from build123d import *

# Parameters (mm, degrees)
BOSS_EXTRUDE1_DEPTH             = 9.525
F_70_0_028_DIAMETER_HOLE1_D     = 0.7112
F_70_0_028_DIAMETER_HOLE1_DEPTH = 2.413
F_70_0_028_DIAMETER_HOLE1_TIP   = 0.213666036
FILLET5_R                       = 6.35
SKETCH90_W                      = 3.175
SKETCH90_H                      = 34.29
CUT_EXTRUDE5_DEPTH              = 49.230860727


with BuildPart() as part:
    # Sketch3 → Boss-Extrude1 (new, symmetric)
    with BuildSketch(Plane.XY):
        Polygon((0, 0), (0, 44.45), (-8.89, 44.45), (-11.43, 44.45), (-11.43, 40.64), (-8.89, 38.1), (-8.89, 16.68503416), (-16.114831723, 4.17125854), (-8.89, 0), align=None)
    extrude(amount=BOSS_EXTRUDE1_DEPTH, both=True)

    # Sketch5 → UPCHURCH 6-32 CONE (revolve, cut)
    with BuildSketch(Plane(origin=(-4.445, 25.259183771, 8.769011984), x_dir=(0, -0.8515022287907943, 0.52435098394521), z_dir=(-1, 0, 0))):
        Polygon((15.292959977, -18.808573968), (15.757749291, -16.067720643), (16.864704876, -14.270117175), (16.687021127, -14.160700376), (16.599421786, -13.998522648), (17.024527056, -14.010579296), (17.217736651, -13.696823041), (17.015625379, -13.322642754), (17.440730649, -13.334699402), (17.633940244, -13.020943147), (17.431828973, -12.64676286), (17.856934243, -12.658819508), (18.050143838, -12.345063253), (17.848032566, -11.970882966), (18.273137836, -11.982939614), (18.466347431, -11.669183359), (18.26423616, -11.295003072), (18.68934143, -11.30705972), (18.498219672, -10.503286273), (20.17440181, -11.535471185), (15.113366113, -19.754170697), (14.821385998, -19.574370744), align=None)
    upchurch_6_32_cone = revolve(axis=Axis((-4.445, 2.032, -2.119740469), (0, 0, 1)), mode=Mode.SUBTRACT)

    # Mirror1: UPCHURCH 6-32 CONE across plane
    add(upchurch_6_32_cone.mirror(Plane.XY), mode=Mode.SUBTRACT)

    # Sketch52 → UPCHURCH 10-32 CONE (revolve, cut)
    with BuildSketch(Plane(origin=(-19.421374868, 2.468387248, 20.886307367), x_dir=(-0.22324939894345092, 0.4655392731409244, -0.8564069657790084), z_dir=(0.47332472697656286, 0.8198224756020795, 0.32226512583622835)), mode=Mode.PRIVATE) as upchurch_10_32_cone_sk:
        Polygon((13.895467161, -20.280398331), (14.632657074, -18.71527204), (14.83876907, -16.459597929), (14.558395769, -16.101111936), (15.153942241, -14.836708527), (15.004691459, -14.766409937), (15.194529151, -14.750538548), (15.345290492, -14.430457474), (15.094342029, -14.069108794), (15.532753397, -14.03245539), (15.683514739, -13.712374317), (15.432566276, -13.351025636), (15.870977644, -13.314372232), (16.021738986, -12.994291159), (15.770790523, -12.632942478), (16.209201891, -12.596289075), (16.359963233, -12.276208001), (16.10901477, -11.914859321), (16.547426138, -11.878205917), (16.698187479, -11.558124844), (16.447239017, -11.196776163), (16.885650385, -11.16012276), (16.460208405, -9.977058466), (19.102754425, -11.221723695), (14.665252306, -20.642974723), align=None)
    revolve(upchurch_10_32_cone_sk.sketch.rotate(Axis((-5.104911358, 2.413, 0), (-0.86602540378444, 0.49999999999999756, 0)), 108.799965538), axis=Axis((-5.104911358, 2.413, 0), (-0.86602540378444, 0.49999999999999756, 0)), mode=Mode.SUBTRACT)

    # #70 (0.028) Diameter Hole1
    with Locations(Plane(origin=(-4.873543168, 2.81374146, 0), x_dir=(0.49999999999999745, 0.86602540378444, 0), z_dir=(-0.8660254037844402, 0.4999999999999975, 0))):
        with Locations((-0.46273638, 0)):
            Hole(F_70_0_028_DIAMETER_HOLE1_D / 2, depth=F_70_0_028_DIAMETER_HOLE1_DEPTH)
            with Locations((0, 0, -(F_70_0_028_DIAMETER_HOLE1_DEPTH + F_70_0_028_DIAMETER_HOLE1_TIP / 2))):  # 118° drill point
                Cone(0, F_70_0_028_DIAMETER_HOLE1_D / 2, F_70_0_028_DIAMETER_HOLE1_TIP, mode=Mode.SUBTRACT)

    # Fillet5
    fillet5_edges = [part.edges().sort_by_distance(p)[0] for p in [
        (-8.89, 16.68503416, 0),
        (-8.89, 38.1, 0),
    ]]
    fillet(fillet5_edges, radius=FILLET5_R)

    # Sketch90 → Cut-Extrude5 (cut, through all)
    with BuildSketch(Plane(origin=(0, 0, 0), x_dir=(0, 0, -1), z_dir=(1, 0, 0))):
        with Locations((-7.9375, 27.305)):
            Rectangle(SKETCH90_W, SKETCH90_H)
        with Locations((7.9375, 27.305)):
            Rectangle(SKETCH90_W, SKETCH90_H)
    extrude(amount=-CUT_EXTRUDE5_DEPTH, mode=Mode.SUBTRACT)


solid = part.part
Design review of the part built by this model. Coordinates are the model's own, in mm. A direction names the side the tool comes from. Coordinates: 2 decimals unless noted, no trailing zeros. Loops run counter-clockwise (first coordinate to the right, second up) from the corner with the lowest first, then second, coordinate; pieces in that order, holes last. Notation, with made-up numbers: (21, 61) - (44, 61) arc R15 cw to (44, 76) - close; hole circle Ø10 at (-11, 50.25). An arc over 180 degrees is marked (long way). Use CSV: the item, a comma, the result in double quotes. Start each with the question number.
1. Add section B-B on z = -4.75. Give the boundary of the cut face in (x, y) (3 decimals).
2. Add section C-C on y = 25. Give the boundary of the cut face in (x, z).
3. For faces 1 (the cylindrical face through (-3.91, 3.31, -5.95)), 2 (the cylindrical face through (-5.96, 2.69, 0.83)), 3 (the flat face through (-6, 10.16, -8)), list the 3-axis set-ups (+Z, -Z, +X, -X, +Y, -Y) from which the entire face can be reached by the end or side of a thin tool; tool diameter is ignored.
4. To check wall thickness, follow probe 1 along X at (y, z) = (4, 0.75); probe 2 along Z at (x, y) = (-5.5, 18.5); probe 3 along X at (y, z) = (18.5, -5). State the ranges of each line that lie inside material, in increasing order.
5. Clearance check with flat-ended pins moving along their axes: pin 1 (8 mm diameter, centred on x = -9.5, z = 1, fed in from -Y); pin 2 (1 mm diameter, centred on x = -4.5, y = 1.5, fed in from +Z); pin 3 (3 mm diameter, centred on x = -4.445, y = 2.032, fed in from +Z); pin 4 (2.5 mm diameter, centred on x = -4.445, y = 2.032, fed in from -Z). State where each tip first meets the part, or that it passes through.
6. Add section A-A on x = -1.5. Give the boundary of the cut face in (y, z) (3 decimals), plus the area to 3 significant figures.
7. Mouldability with a two-part tool opening along Z and no side actions: class faces 4 (the flat face through (-8, 5, -9.525)), 5 (the flat face through (-6, 10.16, 8)), 6 (the cylindrical face through (-10.51, 7.7, 0.78)) as released by +Z, released by -Z, zero draft, split by the parting line, or undercut.
8. Add section D-D on y = 17. Give the boundary of the cut face in (x, z), plus the area to 3 significant figures.
Resolved:
1,outline,"(-16.115, 4.171) - (-8.89, 0) - (0, 0) - (0, 44.45) - (-11.43, 44.45) - (-11.43, 40.64) - (-10.75, 39.96) arc R6.35 cw to (-8.89, 35.47) - (-8.89, 18.387) arc R6.35 cw to (-9.741, 15.212) - close; hole circle Ø2.769 at (-4.445, 2.032)"
2,outline,"(-8.89, -6.35) - (0, -6.35) - (0, 6.35) - (-8.89, 6.35) - close"
3,face 1,"-Z"
3,face 2,"none"
3,face 3,"-Z, +X, -X, +Y"
4,probe 1,"-15.82 to -12.25, -12.07 to -11.63, -6.59 to 0"
4,probe 2,"-6.35 to 6.35"
4,probe 3,"-8.89 to 0"
5,pin 1,"y = 0"
5,pin 2,"z = 2.48"
5,pin 3,"z = 9.06"
5,pin 4,"z = -3.02"
6,outline,"(0, -9.525) - (10.16, -9.525) - (10.16, -6.35) - (44.45, -6.35) - (44.45, 6.35) - (10.16, 6.35) - (10.16, 9.525) - (0, 9.525) - close"
6,area,"629 mm2"
7,face 4,"released by -Z"
7,face 5,"zero draft"
7,face 6,"undercut"
8,outline,"(-9.04, -6.35) - (0, -6.35) - (0, 6.35) - (-9.04, 6.35) - close"
8,area,"115 mm2"
